```python
from build123d import *

# Parameters (mm, degrees)
BOSS_EXTRUDE1_DEPTH  = 57.15
SKETCH1_3_W          = 50.8
SKETCH1_3_H          = 57.15
SKETCH1_3_R          = 1.651
SKETCH1_3_R_2        = 1.5875
BOSS_EXTRUDE2_DEPTH  = 3.175
SKETCH2_R            = 1.651
CUT_EXTRUDE1_DEPTH   = 3.175
FILLET1_R            = 1.5875
FILLET1_OF_MIRROR1_R = 1.5875


with BuildPart() as part:
    # Sketch1 → Boss-Extrude1 (new body)
    with BuildSketch(Plane.XY):
        Polygon((-28.575, 0), (0, 0), (0, 3.175), (-25.4, 3.175), (-25.4, 53.975), (-25.4, 57.15), (-28.575, 57.15), align=None)
    boss_extrude1 = extrude(amount=BOSS_EXTRUDE1_DEPTH)

    # Sketch1<3> → Boss-Extrude2 (add)
    with BuildSketch(Plane.XY):
        with Locations((-53.975, 28.575)):
            Rectangle(SKETCH1_3_W, SKETCH1_3_H)
        with Locations((-53.975, 14.2875)):
            Circle(SKETCH1_3_R, mode=Mode.SUBTRACT)
        with Locations((-53.975, 42.8625)):
            Circle(SKETCH1_3_R_2, mode=Mode.SUBTRACT)
    boss_extrude2 = extrude(amount=BOSS_EXTRUDE2_DEPTH)

    # Sketch2 → Cut-Extrude1 (cut)
    with BuildSketch(Plane.ZY.offset(28.575)):
        with Locations((31.75, 28.575)):
            Circle(SKETCH2_R)
    cut_extrude1 = extrude(amount=-CUT_EXTRUDE1_DEPTH, mode=Mode.SUBTRACT)

    # Fillet1
    fillet1_edges = [part.edges().sort_by_distance(p)[0] for p in [
        (-25.4, 30.1625, 0),
        (-25.4, 3.175, 28.575),
        (-28.575, 0, 30.1625),
        (-28.575, 57.15, 30.1625),
        (-53.975, 0, 3.175),
        (-79.375, 0, 1.5875),
        (-79.375, 57.15, 1.5875),
        (-28.575, 28.575, 3.175),
        (-53.975, 57.15, 3.175),
        (-12.7, 3.175, 0),
    ]]
    fillet(fillet1_edges, radius=FILLET1_R - 0.0001)  # a hair under: the kernel refuses the full size

    # Mirror1: Boss-Extrude1, Boss-Extrude2, Cut-Extrude1 across plane
    add(boss_extrude1.mirror(Plane(origin=(0, 0, 0), x_dir=(0, 0, 1), z_dir=(1, 0, 0))))
    add(boss_extrude2.mirror(Plane(origin=(0, 0, 0), x_dir=(0, 0, 1), z_dir=(1, 0, 0))))
    add(cut_extrude1.mirror(Plane(origin=(0, 0, 0), x_dir=(0, 0, 1), z_dir=(1, 0, 0))), mode=Mode.SUBTRACT)

    # Fillet1 of Mirror1
    fillet1_of_mirror1_edges = [part.edges().sort_by_distance(p)[0] for p in [
        (25.4, 30.1625, 0),
        (25.4, 3.175, 28.575),
        (28.575, 0, 30.1625),
        (28.575, 57.15, 30.1625),
        (53.975, 0, 3.175),
        (79.375, 0, 1.5875),
        (79.375, 57.15, 1.5875),
        (28.575, 28.575, 3.175),
        (53.975, 57.15, 3.175),
        (12.7, 3.175, 0),
    ]]
    fillet(fillet1_of_mirror1_edges, radius=FILLET1_OF_MIRROR1_R - 0.0001)  # a hair under: the kernel refuses the full size


solid = part.part
```
Verification items for the finished model (mm, model axes). A direction names the side the tool comes from. Give positions to 0.01 mm unless a question says otherwise; leave off trailing zeros. Loops run counter-clockwise (first coordinate to the right, second up) from the corner with the lowest first, then second, coordinate; pieces in that order, holes last.
1. Thickness scan on line 1 (X direction, y = 42, z = 19) (3 decimals); line 2 (X direction, y = 19, z = 3) (3 decimals); line 3 (Y direction, x = 26.5, z = 31.75). Record the ranges inside material, lowest first.
2. Go/stop test with flat-tipped pins: pin 1 Ø6 at (y, z) = (28.5, 45.5) entering from +X (3 decimals); pin 2 Ø2 at (x, y) = (58.5, 38.5) entering from +Z (3 decimals); pin 3 Ø3 at (y, z) = (48.5, 28) entering from -X (3 decimals). Record where each tip stops, or that it passes through.
3. Mould release check, pull along Y, two halves, no side actions. Record for faces 1 (the flat face through (-28.575, 29, 36)), 2 (the flat face through (-26, 57.15, 16)), 3 (the cylindrical face through (53.12, 44.2, 1.57)): released by +Y, released by -Y, zero draft, split by the parting line, or undercut.
4. Section check B-B, the plane z = 31.75. Enter the section's corners in (x, y) (3 decimals), then the cut area to 3 significant figures.
5. Set-up check for faces 4 (the flat face through (28.575, 29, 36)), 5 (the flat face through (-55, 29, 3.175)), 6 (the flat face through (0, 3.175, 29)): record each of +Z, -Z, +X, -X, +Y, -Y from which the full face is reachable in a straight line by a thin tool's end or side.
6. Section check A-A, the plane y = 39. Enter the section's corners in (x, z) (3 decimals), then the cut area to 3 significant figures.
7. Section check D-D, the plane x = -11.5. Enter the section's corners in (y, z) (3 decimals).
8. Section check C-C, the plane x = 64. Enter the section's corners in (y, z) (3 decimals), then the cut area to 3 significant figures.
Geometry says:
1. line 1: x = -28.575 to -25.4, 25.4 to 28.575
1. line 2: x = -79.375 to -25.4, 25.4 to 79.375
1. line 3: y = 0 to 26.92, 30.23 to 57.15
2. pin 1: stops at x = 28.575
2. pin 2: stops at z = 3.175
2. pin 3: stops at x = -28.575
3. face 1: zero draft
3. face 2: released by +Y
3. face 3: undercut
4. outline: (-28.575, 1.587) arc R1.587 ccw to (-26.988, 0) - (26.988, 0) arc R1.587 ccw to (28.575, 1.587) - (28.575, 26.924) - (25.4, 26.924) - (25.4, 4.762) arc R1.587 cw to (23.813, 3.175) - (-23.813, 3.175) arc R1.587 cw to (-25.4, 4.762) - (-25.4, 26.924) - (-28.575, 26.924) - close; (-28.575, 30.226) - (-25.4, 30.226) - (-25.4, 57.15) - (-26.988, 57.15) arc R1.587 ccw to (-28.575, 55.563) - close; (25.4, 30.226) - (28.575, 30.226) - (28.575, 55.563) arc R1.587 ccw to (26.988, 57.15) - (25.4, 57.15) - close
4. area: 502 mm2
5. face 4: +Z, +X, +Y, -Y
5. face 5: +Z, -X, +Y, -Y
5. face 6: +Z, -Z, +Y
6. outline: (-79.375, 0) - (-26.987, 0) arc R1.587 ccw to (-25.4, 1.587) - (-25.4, 57.15) - (-28.575, 57.15) - (-28.575, 4.762) arc R1.587 cw to (-30.162, 3.175) - (-79.375, 3.175) - close; (25.4, 1.587) arc R1.587 ccw to (26.987, 0) - (79.375, 0) - (79.375, 3.175) - (30.162, 3.175) arc R1.587 cw to (28.575, 4.762) - (28.575, 57.15) - (25.4, 57.15) - close
6. area: 685 mm2
7. outline: (0, 0) - (1.588, 0) arc R1.587 ccw to (3.175, 1.587) - (3.175, 57.15) - (0, 57.15) - close
8. outline: (0, 0) - (57.15, 0) - (57.15, 1.588) arc R1.587 ccw to (55.563, 3.175) - (1.587, 3.175) arc R1.587 ccw to (0, 1.588) - close
8. area: 180 mm2
